```python
from build123d import *

# Parameters (mm, degrees)
F0_W     = 1050
F0_H     = 378
F0_W_2   = 20.3
F0_H_2   = 3.3
F0_R     = 35
F1_DEPTH = 3


with BuildPart() as f1:
    # F0 (on Top) → F1 (new body)
    with BuildSketch(Plane.XY):
        with Locations((0, -89.869341)):
            Rectangle(F0_W, F0_H)
        with Locations((-485, -115.369341)):
            Rectangle(F0_W_2, F0_H_2, mode=Mode.SUBTRACT)
        with Locations((-242.5, -115.369341)):
            Rectangle(F0_W_2, F0_H_2, mode=Mode.SUBTRACT)
        with Locations((0, -233.869341)):
            Circle(F0_R, mode=Mode.SUBTRACT)
        with Locations((0, -115.369341)):
            Rectangle(F0_W_2, F0_H_2, mode=Mode.SUBTRACT)
        with Locations((242.5, -115.369341)):
            Rectangle(F0_W_2, F0_H_2, mode=Mode.SUBTRACT)
        with Locations((485, -115.369341)):
            Rectangle(F0_W_2, F0_H_2, mode=Mode.SUBTRACT)
        with Locations((-480, 54.130659)):
            Circle(F0_R, mode=Mode.SUBTRACT)
        with Locations((-400, 54.130659)):
            Circle(F0_R, mode=Mode.SUBTRACT)
        with Locations((-320, 54.130659)):
            Circle(F0_R, mode=Mode.SUBTRACT)
        with Locations((-240, 54.130659)):
            Circle(F0_R, mode=Mode.SUBTRACT)
        with Locations((-160, 54.130659)):
            Circle(F0_R, mode=Mode.SUBTRACT)
        with Locations((-80, 54.130659)):
            Circle(F0_R, mode=Mode.SUBTRACT)
        with Locations((0, 54.130659)):
            Circle(F0_R, mode=Mode.SUBTRACT)
        with Locations((80, 54.130659)):
            Circle(F0_R, mode=Mode.SUBTRACT)
        with Locations((160, 54.130659)):
            Circle(F0_R, mode=Mode.SUBTRACT)
        with Locations((240, 54.130659)):
            Circle(F0_R, mode=Mode.SUBTRACT)
        with Locations((320, 54.130659)):
            Circle(F0_R, mode=Mode.SUBTRACT)
        with Locations((400, 54.130659)):
            Circle(F0_R, mode=Mode.SUBTRACT)
        with Locations((480, 54.130659)):
            Circle(F0_R, mode=Mode.SUBTRACT)
    extrude(amount=F1_DEPTH)


solid = f1.part
```
Here's how the part is built. I have some questions about the finished solid (model axes, mm). Round coordinates to 2 decimals unless told otherwise and drop trailing zeros. Loops run counter-clockwise (first coordinate to the right, second up) from the corner with the lowest first, then second, coordinate; pieces in that order, holes last.
1. Suppose I cut it at A-A, the plane x = -400. Please give me the cut outline in (y, z), and give its area (3 significant figures).
Answers:
outline: (-278.87, 0) - (19.13, 0) - (19.13, 3) - (-278.87, 3) - close; (89.13, 0) - (99.13, 0) - (99.13, 3) - (89.13, 3) - close
area: 924 mm2
2. If I drill on probe 1 along Y at (x, z) = (0, 1.3); probe 2 along Y at (x, z) = (403, 0.65); probe 3 along Y at (x, z) = (-320, 2.25), over which ranges is the centre line in solid material (lowest first)?
Answers:
probe 1: y = -278.87 to -268.87, -198.87 to -117.02, -113.72 to 19.13, 89.13 to 99.13
probe 2: y = -278.87 to 19.26, 89 to 99.13
probe 3: y = -278.87 to 19.13, 89.13 to 99.13
3. Suppose I cut it at B-B, the plane x = 307. Please give me the cut outline in (y, z).
Answers:
outline: (-278.87, 0) - (21.63, 0) - (21.63, 3) - (-278.87, 3) - close; (86.63, 0) - (99.13, 0) - (99.13, 3) - (86.63, 3) - close
4. Suppose I cut it at C-C, the plane z = 1.75. Give the number of separate pieces and of enclosed holes in the cut face, and give its area (3 significant figures).
Answers:
separate pieces: 1
enclosed holes: 19
area: 343,000 mm2
5. Thinking about a two-plate mould opening in X: for faces 1 (the face through (-46.616, 64.644, 1.479)), 2 (the face through (-7, -129, 0)), which applies, released by +X, released by -X, zero draft, split by the parting line, or undercut?
Answers:
face 1: undercut
face 2: zero draft
